Work out the finished part from the listing and answer in its coordinate system (mm). A direction names the side the tool comes from. Coordinates: 2 decimals unless noted, no trailing zeros. Order: outer loops, then holes, each group sorted by start corner. A loop starts at its lowest first (then second) coordinate and runs counter-clockwise, first axis right, second up. Notation, with made-up numbers: M -37,79 L 13,79 A29 ccw 13,109 Z; hole C -39.5,12 d2. An arc over 180 degrees is marked long. Write item = value, one per line. Start each with the question number.
Q1. A tool of negligible diameter and unlimited length cuts with its end or side. For faces 1 (the flat face through (2, 15, 5.6)), 2 (the flat face through (19, 0, 5)), from which of +Z, -Z, +X, -X, +Y, -Y can it reach the whole face along a straight path? Write none if from no direction.
Q2. Find section C-C on z = 3.5. Give the vertices of the cut face in (x, y) (3 decimals).
Q3. Each of these flat-tipped pins is pushed along its axis until it touches: P1, Ø5, axis at x = -2, y = 13.5, coming from the -Z side; P2, Ø3, axis at x = -1, y = 11, coming from the -Z side. Where does it stop, or does it pass through?
Q4. Determine the mould class of faces 3 (the cylindrical face through (-11.94, 10.94, 5.03)), 4 (the flat face through (-6, 12, 10.2)), 5 (the flat face through (2, 17, 6)) for opening direction Y: released by +Y, released by -Y, zero draft, split by the parting line, or undercut.
Q5. Find section A-A on y = 0. Give the vertices of the cut face in (x, z).
Q6. Find section B-B on x = 2. Give the vertices of the cut face in (y, z), and give its area (3 significant figures).
Q7. Find section D-D on y = 11.5. Give the vertices of the cut face in (x, z), and give its area (3 significant figures).
Q8. Straight lines are drawn through the part: line 1 along X through (y, z) = (0, 5.5); line 2 along X through (y, z) = (9.5, 7); line 3 along Y through (x, z) = (2, 6.75). For each, find the intervals that lie inside material, in ascending order.
Autodesk Inventor part; units mm, degrees
ref_plane "YZ Plane" through (0, 0, 0) normal (1, 0, 0) x (0, 1, 0)
ref_plane "XZ Plane" through (0, 0, 0) normal (0, 1, 0) x (-1, 0, 0)
ref_plane "XY Plane" through (0, 0, 0) normal (0, 0, 1) x (1, 0, 0)
sketch "Base" plane through (0, 0, 0) normal (0, 0, 1) x (1, 0, 0)
  line L0 (19.0001, -14.9999) -> (19.0001, 15.0001)
  line L1 (19.0001, 15.0001) -> (17.0001, 17.0001)
  line L2 (17.0001, 17.0001) -> (-12.9999, 17.0001)
  line L3 (-12.9999, 17.0001) -> (-14.9999, 15.0001)
  line L4 (-14.9999, 15.0001) -> (-14.9999, -14.9999)
  line L5 (-14.9999, -14.9999) -> (-12.9999, -16.9999)
  line L6 (-12.9999, -16.9999) -> (17.0001, -16.9999)
  line L7 (17.0001, -16.9999) -> (19.0001, -14.9999)
  circle A0 centre (-10.3744, 12.3746) radius 1.75 construction
  circle A1 centre (-2.9999, 8.7501) radius 0.475 construction
  circle A2 centre (-0.4999, 8.7501) radius 0.475 construction
  circle A3 centre (2.0001, 8.7501) radius 0.475 construction
  circle A4 centre (4.5001, 8.7501) radius 0.475 construction
  circle A5 centre (7.0001, 8.7501) radius 0.475 construction
  circle A6 centre (14.3746, 12.3746) radius 1.75 construction
  circle A7 centre (-10.3744, -12.3744) radius 1.75 construction
  circle A8 centre (14.3746, -12.3744) radius 1.75 construction
  line L8 (-5.7099, 9.0001) -> (-5.7099, 16.0001) construction
  line L9 (9.7101, 9.0001) -> (9.7101, 16.0001) construction
  line L10 (-5.7099, 16.0001) -> (9.7101, 16.0001) construction
  circle A9 centre (2, 0) radius 2.5 construction
  circle A10 centre (-10.3744, 12.3746) radius 4 construction
  circle A11 centre (14.3746, 12.3746) radius 4 construction
  circle A12 centre (14.3746, -12.3744) radius 4 construction
  circle A13 centre (-10.3744, -12.3744) radius 4 construction
  line L11 (-6.3744, 12.3746) -> (-6.3744, 17.0001)
  line L12 (10.3746, 12.3746) -> (10.3746, 17.0001)
  circle A14 centre (2, 0) radius 13.5002
  line L13 (-21.7999, 0) -> (25.8001, 0) construction
  line L14 (-6.3744, 12.3746) -> (-6.3744, 10.5889)
  line L15 (10.3746, 12.3746) -> (10.3746, 10.5887)
  circle A15 centre (-10.3744, 12.3746) radius 2.125
  circle A16 centre (-10.3744, -12.3744) radius 2.125
  circle A17 centre (14.3746, -12.3744) radius 2.125
  circle A18 centre (14.3746, 12.3746) radius 2.125
  point P0 (0, 0)
  point P1 (-7.5221, -9.57)
  point P2 (-7.57, -9.5221)
  dimension "d8" = 8
  dimension "d13" = 3.5
  dimension "d14" = 4.25
extrude "BaseFeature" add sketch "Base" along normal blind 10.2 contours L7 L6 L5 L4 L3 L2 L11 L14 A14 L15 L12 L1 L0 | L12 L15 A14 L14 L11 L2
extrude "ConnectorHoleFeature" cut sketch "Base" along normal blind 5.6 contours L12 L15 A14 L14 L11 L2
properties part number "ArmEncoderSpacer"
Findings below:
q1.face_1 = -Z, +Y
q1.face_2 = +Z, -Z, +X, +Y, -Y
q2.outline = M -15,-15 L -13,-17 L 17,-17 L 19,-15 L 19,15 L 17,17 L 10.375,17 L 10.375,10.589 A13.5 cw long -6.374,10.589 L -6.374,17 L -13,17 L -15,15 Z; hole C -10.374,-12.374 d4.25; hole C -10.374,12.375 d4.25; hole C 14.375,-12.374 d4.25; hole C 14.375,12.375 d4.25
q3.P1 = 5.6
q3.P2 = through
q4.face_3 = undercut
q4.face_4 = zero draft
q4.face_5 = released by +Y
q5.outline = M -15,0 L -11.5,0 L -11.5,10.2 L -15,10.2 Z; M 15.5,0 L 19,0 L 19,10.2 L 15.5,10.2 Z
q6.outline = M -17,0 L -13.5,0 L -13.5,10.2 L -17,10.2 Z; M 13.5,5.6 L 17,5.6 L 17,10.2 L 13.5,10.2 Z
q6.area = 51.8 mm^2
q7.outline = M -15,0 L -12.31,0 L -12.31,10.2 L -15,10.2 Z; M -8.44,0 L -6.37,0 L -6.37,5.6 L -5.07,5.6 L -5.07,10.2 L -8.44,10.2 Z; M 9.07,5.6 L 10.37,5.6 L 10.37,0 L 12.44,0 L 12.44,10.2 L 9.07,10.2 Z; M 16.31,0 L 19,0 L 19,10.2 L 16.31,10.2 Z
q7.area = 109 mm^2
q8.line_1 = -15 to -11.5, 15.5 to 19
q8.line_2 = -15 to -7.59, 11.59 to 19
q8.line_3 = -17 to -13.5, 13.5 to 17
